from build123d import *

# Parameters (mm, degrees)
SKETCH1_W           = 92
SKETCH1_H           = 55
SKETCH1_R           = 1.5
BOSS_EXTRUDE3_DEPTH = 2.5
SKETCH4_W           = 55
SKETCH4_H           = 15
BOSS_EXTRUDE4_DEPTH = 10
SKETCH5_W           = 55
SKETCH5_H           = 15
BOSS_EXTRUDE5_DEPTH = 10
SKETCH6_R           = 2.38125
CUT_EXTRUDE1_DEPTH  = 8
CUT_EXTRUDE2_REACH  = 66.166
SKETCH7_R           = 1.190625
CUT_EXTRUDE4_START  = -8
SKETCH8_R           = 2.38125
CUT_EXTRUDE4_DEPTH  = 8
FILLET1_R           = 5


with BuildPart() as part:
    # Sketch1 → Boss-Extrude3 (new, symmetric)
    with BuildSketch(Plane(origin=(0, 0, 0), x_dir=(1, 0, 0), z_dir=(0, 1, 0))):
        Rectangle(SKETCH1_W, SKETCH1_H)
        with Locations(Location((-24, 19.05, 0), (0, 0, 270))):
            Circle(SKETCH1_R, mode=Mode.SUBTRACT)
        with Locations(Location((24, 19.05, 0), (0, 0, 270))):
            Circle(SKETCH1_R, mode=Mode.SUBTRACT)
        with Locations(Location((-24, -19.05, 0), (0, 0, 270))):
            Circle(SKETCH1_R, mode=Mode.SUBTRACT)
        with Locations(Location((24, -19.05, 0), (0, 0, 270))):
            Circle(SKETCH1_R, mode=Mode.SUBTRACT)
    extrude(amount=BOSS_EXTRUDE3_DEPTH, both=True)

    # Sketch4 → Boss-Extrude4 (add)
    with BuildSketch(Plane(origin=(46, 0, 0), x_dir=(0, 0, -1), z_dir=(1, 0, 0))):
        Rectangle(SKETCH4_W, SKETCH4_H)
    extrude(amount=BOSS_EXTRUDE4_DEPTH)

    # Sketch5 → Boss-Extrude5 (add)
    with BuildSketch(Plane.ZY.offset(46)):
        Rectangle(SKETCH5_W, SKETCH5_H)
    extrude(amount=BOSS_EXTRUDE5_DEPTH)

    # Sketch6 → Cut-Extrude1 (cut)
    with BuildSketch(Plane(origin=(56, 0, 0), x_dir=(0, 0, -1), z_dir=(1, 0, 0))):
        Circle(SKETCH6_R)
    extrude(amount=-CUT_EXTRUDE1_DEPTH, mode=Mode.SUBTRACT)

    # Sketch7 → Cut-Extrude2 (cut, up to next)
    with BuildSketch(Plane(origin=(0, 7.5, 0), x_dir=(1, 0, 0), z_dir=(0, 1, 0)), mode=Mode.PRIVATE) as cut_extrude2_sk1:
        with Locations(Location((52, 0, 0), (0, 0, 270))):
            Circle(SKETCH7_R)
    cut_extrude2_tool1 = extrude(cut_extrude2_sk1.sketch, amount=-CUT_EXTRUDE2_REACH, mode=Mode.PRIVATE) & part.part
    # Sketch7 → Cut-Extrude2 (cut, up to next)
    with BuildSketch(Plane(origin=(0, 7.5, 0), x_dir=(1, 0, 0), z_dir=(0, 1, 0)), mode=Mode.PRIVATE) as cut_extrude2_sk2:
        with Locations(Location((-52, 0, 0), (0, 0, 270))):
            Circle(SKETCH7_R)
    cut_extrude2_tool2 = extrude(cut_extrude2_sk2.sketch, amount=-CUT_EXTRUDE2_REACH, mode=Mode.PRIVATE) & part.part
    add(cut_extrude2_tool1.solids().sort_by_distance((52, 7.5, 0))[0], mode=Mode.SUBTRACT)
    add(cut_extrude2_tool2.solids().sort_by_distance((-52, 7.5, 0))[0], mode=Mode.SUBTRACT)

    # Sketch8 → Cut-Extrude4 (cut)
    with BuildSketch(Plane.ZY.offset(56).offset(CUT_EXTRUDE4_START)):
        with Locations(Location((0, 0, 0), (0, 0, 180))):
            Circle(SKETCH8_R)
    extrude(amount=CUT_EXTRUDE4_DEPTH, mode=Mode.SUBTRACT)

    # Fillet1
    fillet1_edges = [part.edges().sort_by_distance(p)[0] for p in [
        (-46, -2.5, 0),
        (46, -2.5, 0),
        (46, 2.5, 0),
        (-46, 2.5, 0),
    ]]
    fillet(fillet1_edges, radius=FILLET1_R - 0.0001)  # a hair under: the kernel refuses the full size


solid = part.part
Design review of the part built by this model. Coordinates are the model's own, in mm. A direction names the side the tool comes from. Round coordinates to 2 decimals unless told otherwise and drop trailing zeros. Loops run counter-clockwise (first coordinate to the right, second up) from the corner with the lowest first, then second, coordinate; pieces in that order, holes last. Notation, with made-up numbers: (-23, 86.5) - (35, 86.5) arc R28 ccw to (35, 104.5) - close; hole circle Ø1 at (-25.5, 30.25). An arc over 180 degrees is marked (long way). One line per item, written item: value. Start each with the question number.
1) Consider section D-D on x = -24. Give the boundary of the cut face in (y, z).
2) Draft analysis for pull direction X (two halves, no side actions). For faces 4 (the flat face through (50, 7.5, 0)), 5 (the cylindrical face through (25.487, -0.035, 18.855)), 6 (the flat face through (-48, 0, 0)), state which applies: +X half, -X half, draft (parallel to the pull), parting line (faces both ways), or undercut.
3) To check wall thickness, follow L1, parallel to X at y = 0.5, z = 19; L2, parallel to X at y = 3.45, z = 0; L3, parallel to X at y = -5, z = 0. State the ranges of each line that lie inside material, in increasing order. Write a range as from..to.
4) Insertion check: pin 1 Ø5 at (x, z) = (-18, -1) entering from +Y; pin 2 Ø4 at (x, z) = (-39, 18) entering from -Y; pin 3 Ø4.5 at (y, z) = (0, 0) entering from -X. Each pin has a flat end and moves straight along its axis. Give the tip position at first contact, or say it passes through.
5) Consider section C-C on y = -6.25. Give the boundary of the cut face in (x, z), then the cut area to 3 significant figures.
6) Consider section B-B on z = 19.05. Give the number of separate pieces and of enclosed holes in the cut face, then the cut area to 3 significant figures.
7) For faces 1 (the flat face through (48, 0, 0)), 2 (the flat face through (-1, 2.5, 0)), 3 (the cylindrical face through (50.84, 4.82, -0.26)), list the 3-axis set-ups (+Z, -Z, +X, -X, +Y, -Y) from which the entire face can be reached by the end or side of a thin tool; tool diameter is ignored.
8) Consider section A-A on x = -52. Give the boundary of the cut face in (y, z).
Reported:
1. outline: (-2.5, -27.5) - (2.5, -27.5) - (2.5, -20.55) - (-2.5, -20.55) - close; (-2.5, -17.55) - (2.5, -17.55) - (2.5, 17.55) - (-2.5, 17.55) - close; (-2.5, 20.55) - (2.5, 20.55) - (2.5, 27.5) - (-2.5, 27.5) - close
2. face 4: draft
2. face 5: undercut
2. face 6: -X half
3. L1: x = -56..-25.5, -22.5..22.5, 25.5..56
3. L2: x = -56..-53.19, -50.81..-43.93, 43.93..50.81, 53.19..56
3. L3: x = -56..-53.19, -50.81..-45.33, 45.33..56
4. pin 1: stops at y = 2.5
4. pin 2: stops at y = -2.5
4. pin 3: stops at x = -48
5. outline: (-56, -27.5) - (-45.84, -27.5) - (-45.84, 27.5) - (-56, 27.5) - close; (45.84, -27.5) - (56, -27.5) - (56, 27.5) - (45.84, 27.5) - close; hole circle Ø2.38 at (-52, 0)
5. area: 1,110 mm^2
6. separate pieces: 3
6. enclosed holes: 0
6. area: 751 mm^2
7. face 1: +X
7. face 2: +Z, -Z, +Y
7. face 3: +Y
8. outline: (-7.5, -27.5) - (7.5, -27.5) - (7.5, -1.19) - (2.06, -1.19) arc R2.38 cw to (-2.06, -1.19) - (-7.5, -1.19) - close; (-7.5, 1.19) - (-2.06, 1.19) arc R2.38 cw to (2.06, 1.19) - (7.5, 1.19) - (7.5, 27.5) - (-7.5, 27.5) - close
